from build123d import *

# Parameters (mm, degrees)
SKETCH2_R           = 2
BOSS_EXTRUDE1_DEPTH = 32
SKETCH11_R          = 1
CUT_EXTRUDE3_DEPTH  = 5
SCALE1_SCALE        = 2


with BuildPart() as part:
    # Sketch2 → Boss-Extrude1 (new body)
    with BuildSketch(Plane(origin=(0, 0, 0), x_dir=(1, 0, 0), z_dir=(0, 1, 0))):
        with Locations(Location((0, 0, 0), (0, 0, 270))):
            Circle(SKETCH2_R)
    extrude(amount=BOSS_EXTRUDE1_DEPTH)

    # Sketch11 → Cut-Extrude3 (cut)
    with BuildSketch(Plane(origin=(0, 32, 0), x_dir=(1, 0, 0), z_dir=(0, 1, 0))):
        with Locations(Location((0, 0, 0), (0, 0, 270))):
            Circle(SKETCH11_R)
    extrude(amount=-CUT_EXTRUDE3_DEPTH, mode=Mode.SUBTRACT)


with BuildPart() as part_1:
    # Scale1: scaled about (0, 0, 0)
    add(part.part.scale(SCALE1_SCALE))


solid = part_1.part
The listing builds one solid part. Answer for the finished solid, in the listing's coordinates (mm). A direction names the side the tool comes from. Give positions to 0.01 mm unless a question says otherwise; leave off trailing zeros. Order: outer loops, then holes, each group sorted by start corner. A loop starts at its lowest first (then second) coordinate and runs counter-clockwise, first axis right, second up. Notation, with made-up numbers: (69, -30.75) -> (78, -30.75) arc R34 cw to (78, 2.25) -> close; hole circle Ø7 at (6.25, 22). An arc over 180 degrees is marked (long way). Put each result on its own line as item: value.
Item 1: For faces 4 (the face through (-1, 64, -2)), 5 (the face through (0, 54, 0)), determine the directions among +Z, -Z, +X, -X, +Y, -Y from which every point of the face is accessible in a straight line to the end or side of a thin tool.
Established:
face 4: +Z, -Z, +X, -X, +Y
face 5: +Y
Item 2: For a pull along Z with two mould halves and no side action, classify faces 1 (the face through (-2, 59, 0)), 2 (the face through (-3.905, 31.552, -0.867)), 3 (the face through (0, 0, 0)) as released by +Z, released by -Z, zero draft, split by the parting line, or undercut.
Established:
face 1: undercut
face 2: split by the parting line
face 3: zero draft
Item 3: A cutting plane is placed at C-C on y = 55. Give the vertices of the cut face in (x, z), plus the area to 3 significant figures.
Established:
outline: circle Ø8 at (0, 0); hole circle Ø4 at (0, 0)
area: 37.7 mm^2
Item 4: A cutting plane is placed at B-B on x = 0. Give the vertices of the cut face in (y, z).
Established:
outline: (0, -4) -> (64, -4) -> (64, -2) -> (54, -2) -> (54, 2) -> (64, 2) -> (64, 4) -> (0, 4) -> close
Item 5: A cutting plane is placed at A-A on z = 0. Give the vertices of the cut face in (x, y).
Established:
outline: (-4, 0) -> (4, 0) -> (4, 64) -> (2, 64) -> (2, 54) -> (-2, 54) -> (-2, 64) -> (-4, 64) -> close
Item 6: Straight lines are drawn through the part: line 1 (X direction, y = 56, z = 0); line 2 (X direction, y = 55, z = 1.25); line 3 (Y direction, x = 1, z = 0.5). For each, find the intervals that lie inside material, in ascending order.
Established:
line 1: x = -4 to -2, 2 to 4
line 2: x = -3.8 to -1.56, 1.56 to 3.8
line 3: y = 0 to 54
Item 7: Given P1, Ø1.2, axis at x = 0, z = -1, coming from the +Y side, flat-ended and moving along its own axis, determine where the tip first touches the part or whether it passes through.
Established:
P1: stops at y = 54
Item 8: A cutting plane is placed at D-D on y = 23. Give the vertices of the cut face in (x, z), plus the area to 3 significant figures.
Established:
outline: circle Ø8 at (0, 0)
area: 50.3 mm^2
